```python
from build123d import *

# Parameters (mm, degrees)
EXTRUDE_1_DEPTH     = 30
SKETCH_2_R          = 15
EXTRUDE_2_DEPTH     = 15
SKETCH_3_R          = 12.5
CUT_EXTRUDE_1_DEPTH = 7


with BuildPart() as part:
    # 草图1 → 凸台-拉伸1 (new body)
    with BuildSketch(Plane.XY):
        with BuildLine():
            Line((-10, -20), (10, -20))
            ThreePointArc((10, -20), (17.071067812, -17.071067812), (20, -10))
            Line((20, -10), (20, 10))
            ThreePointArc((20, 10), (17.071067812, 17.071067812), (10, 20))
            Line((10, 20), (-10, 20))
            ThreePointArc((-10, 20), (-17.071067812, 17.071067812), (-20, 10))
            Line((-20, 10), (-20, -10))
            ThreePointArc((-20, -10), (-17.071067812, -17.071067812), (-10, -20))
        make_face()
    extrude(amount=-EXTRUDE_1_DEPTH)

    # 草图2 → 凸台-拉伸2 (add)
    with BuildSketch(Plane.XY):
        Circle(SKETCH_2_R)
    extrude(amount=EXTRUDE_2_DEPTH)

    # 草图3 → 切除-拉伸1 (cut)
    with BuildSketch(Plane.XY.offset(15)):
        Circle(SKETCH_3_R)
    extrude(amount=-CUT_EXTRUDE_1_DEPTH, mode=Mode.SUBTRACT)

    # 草图4 → 旋转1 (revolve)
    with BuildSketch(Plane(origin=(0, 0, 0), x_dir=(1, 0, 0), z_dir=(0, 1, 0))):
        with BuildLine():
            Line((0, -8), (12.5, -8))
            add(Edge.make_bspline(
                [(0, -14), (2.433971775, -14.017624523), (6.926016956, -12.41143597), (11.019102747, -9.936800199), (12.5, -8)],
                knots=[0, 0, 0, 0, 0.499949421, 1, 1, 1, 1], degree=3))
            Line((0, -14), (0, -8))
        make_face()
    revolve(axis=Axis((0, 0, 20.621681052), (0, 0, -1)))


solid = part.part
```
CAD build for the part. Positions are in the model's coordinates, mm. A direction names the side the tool comes from. Round coordinates to 2 decimals unless told otherwise and drop trailing zeros. Write each loop counter-clockwise with the first axis right and the second up, starting at its lowest first coordinate (ties: lowest second). Pieces come first, ordered by that corner, then holes. Notation, with made-up numbers: (-22.75, 10.5) -> (-17.75, 10.5) arc R21 cw to (-17.75, 31.5) -> close; hole circle Ø8 at (-23, 42.5). An arc over 180 degrees is marked (long way). Answer in a Markdown table with one row per item. Add a question column.
Item 1: Saw through at A-A, the plane z = -16. Write the cut outline in (x, y).
Item 2: Which spindle directions (+Z, -Z, +X, -X, +Y, -Y) get a long thin tool onto all of the face, cutting with end or side? Do faces 5 (the face through (9, 14, 0)), 6 (the face through (0, 0, -30)). Say none if no direction does.
Item 3: Saw through at B-B, the plane x = -13.5. Write the cut outline in (y, z).
Item 4: Drop flat-ended pins along their axis: pin 1 Ø4 at (y, z) = (13.5, 9) entering from -X; pin 2 Ø15 at (x, y) = (0, 0) entering from +Z. Give the stop position or say it passes through.
Item 5: Drill centre lines: line 1 (Y direction, x = 0, z = 11.25); line 2 (X direction, y = -4.5, z = 11); line 3 (Z direction, x = 14.5, y = 5.5). Where is each one in solid material? Low to high. Write a range as from..to.
Item 6: Mould opens along X. For faces 1 (the face through (-14.985, 0.66, 7.395)), 2 (the face through (11.923, 3.755, 11.549)), 3 (the face through (-16.99, 17.15, -14.79)), 4 (the face through (20, 0, -15)) say: pulls with the +X half, pulls with the -X half, needs draft (parallel to the pull), parting line crosses it, or undercut.
Findings below:
| question | item | result |
|---|---|---|
| 1 | outline | (-20, -10) arc R10 ccw to (-10, -20) -> (10, -20) arc R10 ccw to (20, -10) -> (20, 10) arc R10 ccw to (10, 20) -> (-10, 20) arc R10 ccw to (-20, 10) -> close |
| 2 | face 5 | +Z |
| 2 | face 6 | -Z, +X, -X, +Y, -Y |
| 3 | outline | (-19.37, -30) -> (19.37, -30) -> (19.37, 0) -> (6.54, 0) -> (6.54, 15) -> (-6.54, 15) -> (-6.54, 0) -> (-19.37, 0) -> close |
| 4 | pin 1 | stops at x = -9.63 |
| 4 | pin 2 | stops at z = 14 |
| 5 | line 1 | y = -15..-12.5, -8.64..8.64, 12.5..15 |
| 5 | line 2 | x = -14.31..-11.66, -7.86..7.86, 11.66..14.31 |
| 5 | line 3 | z = -30..0 |
| 6 | face 1 | parting line crosses it |
| 6 | face 2 | undercut |
| 6 | face 3 | pulls with the -X half |
| 6 | face 4 | pulls with the +X half |
